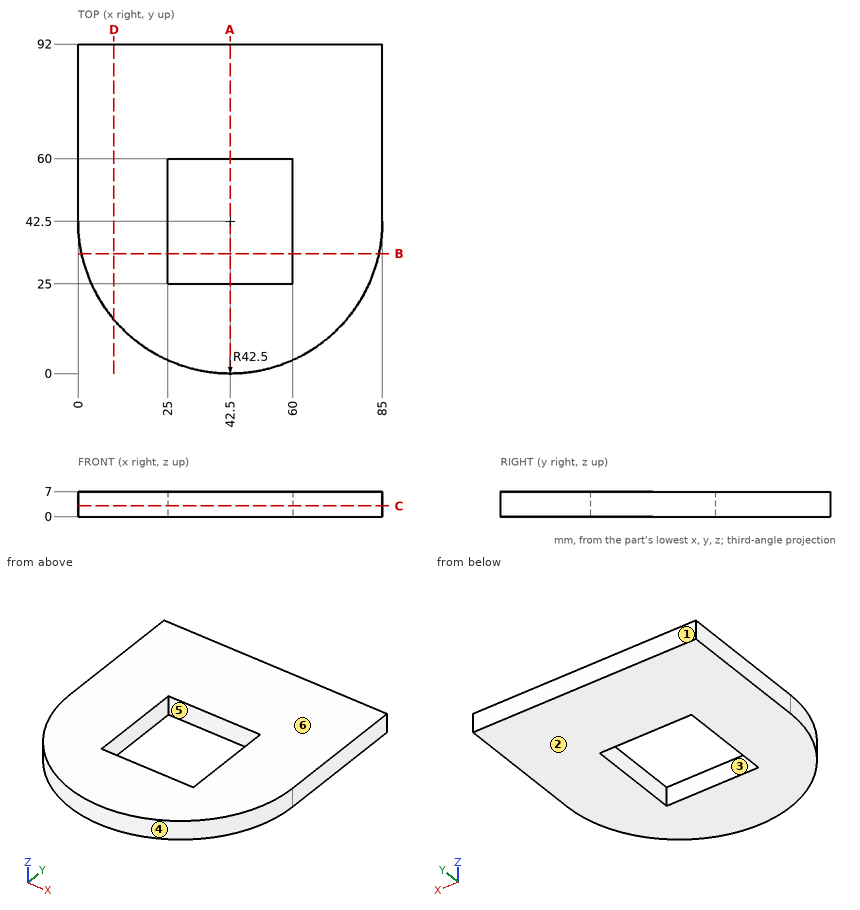
Input: dimensioned drawing with shaded views. Units: mm. Origin: part minimum x, y, z. A direction names the side the tool comes from. Coordinates: 2 decimals unless noted, no trailing zeros. Order: outer loops, then holes, each group sorted by start corner. A loop starts at its lowest first (then second) coordinate and runs counter-clockwise, first axis right, second up.
(1) Draft query along Y for the marked faces 1, 2, 3 and 4. Return one class per face: pulls with the +Y half, pulls with the -Y half, needs draft (parallel to the pull), parting line crosses it, or undercut.
(2) Section query A-A (x = 42.5). Return the cut outline in (y, z).
(3) First-contact query: pin 1 (3 mm diameter, centred on y = 13.5, z = 4.5, fed in from +X); pin 2 (3.5 mm diameter, centred on x = 48, z = 4, fed in from -Y); pin 3 (4 mm diameter, centred on y = 27, z = 3.5, fed in from -X). Flat tips, straight axial feed; report the tip coordinate or a pass-through.
(4) Section query B-B (y = 33.5). Return the cut outline in (x, z).
(5) Access query for the marked faces 5 and 6. Directions: +Z, -Z, +X, -X, +Y, -Y. A direction counts if a zero-diameter tool reaches every point of the face in a straight line with its end or side. Return the directions, or none.
(6) Section query D-D (x = 10). Return the cut outline in (y, z), plus the area to 3 significant figures.
(7) Material intervals for probe 1 along X at (y, z) = (43, 4); probe 2 along Y at (x, z) = (55, 3); probe 3 along Y at (x, z) = (45, 1.5), sorted ascending.
(8) Section query C-C (z = 3). Return the cut outline in (x, y).
Solution:
1. face 1: pulls with the +Y half
1. face 2: needs draft
1. face 3: undercut
1. face 4: pulls with the -Y half
2. outline: (0, 0) - (25, 0) - (25, 7) - (0, 7) - close; (60, 0) - (92, 0) - (92, 7) - (60, 7) - close
3. pin 1: stops at x = 74.9
3. pin 2: stops at y = 0.17
3. pin 3: stops at x = 2.2
4. outline: (0.96, 0) - (25, 0) - (25, 7) - (0.96, 7) - close; (60, 0) - (84.04, 0) - (84.04, 7) - (60, 7) - close
5. face 5: +Z, -Z
5. face 6: +Z, +X, -X, +Y, -Y
6. outline: (15.11, 0) - (92, 0) - (92, 7) - (15.11, 7) - close
6. area: 538 mm2
7. probe 1: x = 0 to 25, 60 to 85
7. probe 2: y = 1.88 to 25, 60 to 92
7. probe 3: y = 0.07 to 25, 60 to 92
8. outline: (0, 42.5) arc R42.5 ccw to (85, 42.5) - (85, 92) - (0, 92) - close; hole (25, 25) - (60, 25) - (60, 60) - (25, 60) - close
